Work out the finished part from the listing and answer in its coordinate system (mm). A direction names the side the tool comes from. Give positions to 0.01 mm unless a question says otherwise; leave off trailing zeros. Order: outer loops, then holes, each group sorted by start corner. A loop starts at its lowest first (then second) coordinate and runs counter-clockwise, first axis right, second up. Notation, with made-up numbers: M -32,51.25 L -23,51.25 A12 cw -23,57.25 Z; hole C 26.25,42 d9. An arc over 180 degrees is marked long. One line per item, written item: value.
from build123d import *

# Parameters (mm, degrees)
SKETCH1_W                 = 140
SKETCH1_H                 = 100
BOSS_EXTRUDE1_DEPTH       = 3
SKETCH3_W                 = 16
SKETCH3_H                 = 100
BOSS_EXTRUDE2_DEPTH       = 2.5
SKETCH4_W                 = 12.2
SKETCH4_H                 = 5.5
CUT_EXTRUDE1_DEPTH        = 1.5
LPATTERN1_COUNT           = 4
LPATTERN1_PITCH           = 30
LPATTERN1_COPY_1_SKETCH_W = 12.2
LPATTERN1_COPY_1_SKETCH_H = 5.5
LPATTERN1_COPY_1_DEPTH    = 1.5
LPATTERN1_COPY_2_SKETCH_W = 12.2
LPATTERN1_COPY_2_SKETCH_H = 5.5
LPATTERN1_COPY_2_DEPTH    = 1.5
LPATTERN1_COPY_3_SKETCH_W = 12.2
LPATTERN1_COPY_3_SKETCH_H = 5.5
LPATTERN1_COPY_3_DEPTH    = 1.5
CUT_EXTRUDE3_DEPTH        = 123.102416029
CUT_EXTRUDE3_DEPTH_BACK   = 123.102416029
SKETCH6_W                 = 0.2
SKETCH6_H                 = 3
CUT_EXTRUDE5_DEPTH        = 1.5
LPATTERN2_COUNT           = 2
LPATTERN2_PITCH           = 30
LPATTERN2_COL_COUNT       = 2
LPATTERN2_COL_PITCH       = 30
MIRROR4_COPY_1_DEPTH      = 1.5
MIRROR4_COPY_2_DEPTH      = 1.5
SKETCH13_W                = 1
SKETCH13_H                = 40
SKETCH13_H_2              = 36
CUT_EXTRUDE7_DEPTH        = 10
SKETCH15_W                = 80
SKETCH15_H                = 3
BOSS_EXTRUDE4_DEPTH       = 10
FILLET2_R                 = 5
FILLET3_R                 = 3
SKETCH17_W                = 12.2
SKETCH17_H                = 2.25
CUT_EXTRUDE9_DEPTH        = 1.5
SKETCH18_R                = 1.6
CUT_EXTRUDE10_DEPTH       = 10


with BuildPart() as part:
    # Sketch1 → Boss-Extrude1 (new body)
    with BuildSketch(Plane.XY):
        Rectangle(SKETCH1_W, SKETCH1_H)
    extrude(amount=BOSS_EXTRUDE1_DEPTH)

    # Sketch3 → Boss-Extrude2 (add)
    with BuildSketch(Plane(origin=(0, 0, 0), x_dir=(-1, 0, 0), z_dir=(0, 0, -1))):
        with Locations((-60, 0)):
            Rectangle(SKETCH3_W, SKETCH3_H)
        with Locations((60, 0)):
            Rectangle(SKETCH3_W, SKETCH3_H)
    extrude(amount=BOSS_EXTRUDE2_DEPTH)

    # Sketch4 → Cut-Extrude1 (cut)
    with BuildSketch(Plane(origin=(0, 0, -2.5), x_dir=(-1, 0, 0), z_dir=(0, 0, -1))):
        with Locations((-60, 45)):
            Rectangle(SKETCH4_W, SKETCH4_H)
    cut_extrude1 = extrude(amount=-CUT_EXTRUDE1_DEPTH, mode=Mode.SUBTRACT)

    # Mirror1: Cut-Extrude1 across plane
    add(cut_extrude1.mirror(Plane(origin=(0, 0, 0), x_dir=(0, 0, 1), z_dir=(1, 0, 0))), mode=Mode.SUBTRACT)

    # LPattern1: Cut-Extrude1 ×4
    with Locations(*[(0, -i * LPATTERN1_PITCH, 0) for i in range(1, LPATTERN1_COUNT)]):
        add(cut_extrude1, mode=Mode.SUBTRACT)

    # LPattern1 copy 1 sketch → LPattern1 copy 1 (cut)
    with BuildSketch(Plane(origin=(0, -30, -2.5), x_dir=(1, 0, 0), z_dir=(0, 0, -1))):
        with Locations((-60, -45)):
            Rectangle(LPATTERN1_COPY_1_SKETCH_W, LPATTERN1_COPY_1_SKETCH_H)
    extrude(amount=-LPATTERN1_COPY_1_DEPTH, mode=Mode.SUBTRACT)

    # LPattern1 copy 2 sketch → LPattern1 copy 2 (cut)
    with BuildSketch(Plane(origin=(0, -60, -2.5), x_dir=(1, 0, 0), z_dir=(0, 0, -1))):
        with Locations((-60, -45)):
            Rectangle(LPATTERN1_COPY_2_SKETCH_W, LPATTERN1_COPY_2_SKETCH_H)
    extrude(amount=-LPATTERN1_COPY_2_DEPTH, mode=Mode.SUBTRACT)

    # LPattern1 copy 3 sketch → LPattern1 copy 3 (cut)
    with BuildSketch(Plane(origin=(0, -90, -2.5), x_dir=(1, 0, 0), z_dir=(0, 0, -1))):
        with Locations((-60, -45)):
            Rectangle(LPATTERN1_COPY_3_SKETCH_W, LPATTERN1_COPY_3_SKETCH_H)
    extrude(amount=-LPATTERN1_COPY_3_DEPTH, mode=Mode.SUBTRACT)

    # Sketch6 → Cut-Extrude3 (cut, two sides: drawn at the far end of the back side and taken through both)
    with BuildSketch(Plane(origin=(0, 50, 0), x_dir=(1, 0, 0), z_dir=(0, 1, 0)).offset(-CUT_EXTRUDE3_DEPTH_BACK)):
        with Locations((-69.9, -1.5)):
            Rectangle(SKETCH6_W, SKETCH6_H)
        with Locations((69.9, -1.5)):
            Rectangle(SKETCH6_W, SKETCH6_H)
    extrude(amount=CUT_EXTRUDE3_DEPTH + CUT_EXTRUDE3_DEPTH_BACK, mode=Mode.SUBTRACT)

    # Sketch11 → Cut-Extrude5 (cut)
    with BuildSketch(Plane(origin=(0, 0, -2.5), x_dir=(-1, 0, 0), z_dir=(0, 0, -1))):
        Polygon((-53.9, 12.25), (-60, -7.75), (-66.1, 12.25), align=None)
    cut_extrude5 = extrude(amount=-CUT_EXTRUDE5_DEPTH, mode=Mode.SUBTRACT)

    # LPattern2: Cut-Extrude5 ×2
    with Locations(*[(0, i * LPATTERN2_PITCH, 0) for i in range(1, LPATTERN2_COUNT)]):
        add(cut_extrude5, mode=Mode.SUBTRACT)

    # LPattern2 col: Cut-Extrude5 ×2
    with Locations(*[(0, -i * LPATTERN2_COL_PITCH, 0) for i in range(1, LPATTERN2_COL_COUNT)]):
        add(cut_extrude5, mode=Mode.SUBTRACT)

    # Mirror4: Cut-Extrude5 across plane
    add(cut_extrude5.mirror(Plane(origin=(0, 0, 0), x_dir=(0, 0, 1), z_dir=(1, 0, 0))), mode=Mode.SUBTRACT)

    # Mirror4 copy 1 sketch → Mirror4 copy 1 (cut)
    with BuildSketch(Plane(origin=(0, 30, -2.5), x_dir=(1, 0, 0), z_dir=(0, 0, -1))):
        Polygon((-53.9, -12.25), (-60, 7.75), (-66.1, -12.25), align=None)
    extrude(amount=-MIRROR4_COPY_1_DEPTH, mode=Mode.SUBTRACT)

    # Mirror4 copy 2 sketch → Mirror4 copy 2 (cut)
    with BuildSketch(Plane(origin=(0, -30, -2.5), x_dir=(1, 0, 0), z_dir=(0, 0, -1))):
        Polygon((-53.9, -12.25), (-60, 7.75), (-66.1, -12.25), align=None)
    extrude(amount=-MIRROR4_COPY_2_DEPTH, mode=Mode.SUBTRACT)

    # Sketch13 → Cut-Extrude7 (cut)
    with BuildSketch(Plane(origin=(0, 0, 0), x_dir=(-1, 0, 0), z_dir=(0, 0, -1))):
        with Locations((-46.5, 25)):
            Rectangle(SKETCH13_W, SKETCH13_H)
        with Locations((-46.5, -23)):
            Rectangle(SKETCH13_W, SKETCH13_H_2)
    cut_extrude7 = extrude(amount=-CUT_EXTRUDE7_DEPTH, mode=Mode.SUBTRACT)

    # Mirror7: Cut-Extrude7 across plane
    add(cut_extrude7.mirror(Plane(origin=(0, 0, 0), x_dir=(0, 0, 1), z_dir=(1, 0, 0))), mode=Mode.SUBTRACT)

    # Sketch15 → Boss-Extrude4 (add)
    with BuildSketch(Plane(origin=(0, 0, 0), x_dir=(-1, 0, 0), z_dir=(0, 0, -1))):
        with Locations((0, 48.5)):
            Rectangle(SKETCH15_W, SKETCH15_H)
    extrude(amount=BOSS_EXTRUDE4_DEPTH)

    # Fillet2
    fillet2_edges = [part.edges().sort_by_distance(p)[0] for p in [
        (40, 48.5, -10),
        (-40, 48.5, -10),
    ]]
    fillet(fillet2_edges, radius=FILLET2_R)

    # Fillet3
    fillet3_edges = [part.edges().sort_by_distance(p)[0] for p in [
        (0, 47, 0),
    ]]
    fillet(fillet3_edges, radius=FILLET3_R)

    # Sketch17 → Cut-Extrude9 (cut)
    with BuildSketch(Plane(origin=(0, 0, -2.5), x_dir=(-1, 0, 0), z_dir=(0, 0, -1))):
        with Locations((-60, -48.875)):
            Rectangle(SKETCH17_W, SKETCH17_H)
    cut_extrude9 = extrude(amount=-CUT_EXTRUDE9_DEPTH, mode=Mode.SUBTRACT)

    # Mirror8: Cut-Extrude9 across plane
    add(cut_extrude9.mirror(Plane(origin=(0, 0, 0), x_dir=(0, 0, 1), z_dir=(1, 0, 0))), mode=Mode.SUBTRACT)

    # Sketch18 → Cut-Extrude10 (cut)
    with BuildSketch(Plane(origin=(0, 50, 0), x_dir=(1, 0, 0), z_dir=(0, 1, 0))):
        with Locations(Location((-25, 3, 0), (0, 0, 180))):
            Circle(SKETCH18_R)
        with Locations(Location((25, 3, 0), (0, 0, 180))):
            Circle(SKETCH18_R)
    extrude(amount=-CUT_EXTRUDE10_DEPTH, mode=Mode.SUBTRACT)


solid = part.part
(1) Section B-B, the plane x = -10 is taken. Give the vertices of the cut face in (y, z), then the cut area to 3 significant figures.
Findings:
outline: M -50,0 L 44,0 A3 cw 47,-3 L 47,-10 L 50,-10 L 50,3 L -50,3 Z
area: 332 mm^2
(2) Section D-D, the plane z = -6.75 is taken. Give the vertices of the cut face in (x, y).
Findings:
outline: M -39.68,47 L 39.68,47 L 39.68,50 L -39.68,50 Z
(3) Which of the six approach directions +Z, -Z, +X, -X, +Y, -Y give full straight-line access (tool end or side, diameter ignored) to faces 4 (the flat face through (46, -23, 1)), 5 (the flat face through (69.8, -1, 2)), 6 (the flat face through (-60, -46, -1)), 7 (the flat face through (60, 8, -1)), 8 (the flat face through (40, 48, -2))?
Findings:
face 4: +Z, -Z
face 5: +Z, -Z, +X, +Y, -Y
face 6: -Z, -Y
face 7: -Z
face 8: -Z, +Y, -Y
(4) Given P1, Ø17.5, axis at x = 62, y = -4.5, coming from the -Z side; P2, Ø0.5, axis at x = 69, y = 18.5, coming from the -Z side; P3, Ø4, axis at x = 25, z = -3, coming from the -Y side; P4, Ø5, axis at x = 49, z = -4, coming from the -Y side, each flat-ended and moving along its own axis, determine where each tip first touches the part or whether it passes through.
Findings:
P1: stops at z = -2.5
P2: stops at z = 0
P3: stops at y = 46.24
P4: passes through
(5) Section C-C, the plane y = 0 is taken. Give the vertices of the cut face in (x, z).
Findings:
outline: M -69.8,0 L -68,0 L -68,-2.5 L -62.36,-2.5 L -62.36,-1 L -57.64,-1 L -57.64,-2.5 L -52,-2.5 L -52,0 L 52,0 L 52,-2.5 L 57.64,-2.5 L 57.64,-1 L 62.36,-1 L 62.36,-2.5 L 68,-2.5 L 68,0 L 69.8,0 L 69.8,3 L -69.8,3 Z
(6) Find the intervals of material crossed by probe 1 along X at (y, z) = (26, 2.5); probe 2 along X at (y, z) = (-41.5, -1); probe 3 along Z at (x, y) = (41, 24), in increasing order. Write a range as from..to.
Findings:
probe 1: x = -69.8..-47, -46..46, 47..69.8
probe 2: x = -68..-52, 52..68
probe 3: z = 0..3
(7) Determine the mould class of faces 1 (the flat face through (-40, 48, -2)), 2 (the flat face through (-60, 8, -1)), 3 (the flat face through (-1, 50, -2)) for opening direction Y: pulls with the +Y half, pulls with the -Y half, needs draft (parallel to the pull), parting line crosses it, or undercut.
Findings:
face 1: needs draft
face 2: undercut
face 3: pulls with the +Y half
(8) Section A-A, the plane x = 25 is taken. Give the vertices of the cut face in (y, z), then the cut area to 3 significant figures.
Findings:
outline: M -50,0 L 44,0 A3 cw 46.54,-1.4 L 50,-1.4 L 50,3 L -50,3 Z; M 47,-10 L 50,-10 L 50,-4.6 L 47,-4.6 Z
area: 322 mm^2
